Autodesk Fusion 360 part; units mm, degrees
sketch "Sketch1" plane through (0, 0, 0) normal (0, 0, 1) x (1, 0, 0)
  line L0 (-50, 25) -> (7.7, 25)
  line L1 (7.7, 25) -> (7.7, 7.3)
  line L2 (7.7, 7.3) -> (-50, 7.3)
  line L3 (-50, 7.3) -> (-50, 25)
  line L4 (6.7, 8.3) -> (-49, 8.3)
  line L5 (-49, 8.3) -> (-49, 24)
  line L6 (-49, 24) -> (6.7, 24)
  line L7 (6.7, 24) -> (6.7, 8.3)
  line L8 (6.7, 8.3) -> (-49, 24) construction
  line L9 (-49, 8.3) -> (6.7, 24) construction
  point P0 (-21.15, 16.15)
  dimension "d1" = 57.7
  dimension "d2" = 17.7
  dimension "d3" = 55.7
  dimension "d4" = 15.7
extrude "Extrude1" add sketch "Sketch1" along normal blind 2 contours L4 L5 L6 L7
extrude "Extrude2" add sketch "Sketch1" along normal blind 13
fillet "Fillet1" radius 2 4 edges at (7.7, 7.3, 6.5) (7.7, 25, 6.5) (-50, 7.3, 6.5) (-50, 25, 6.5)
fillet "Fillet2" radius 2 8 edges at (7.1142, 7.8858, 0) (-21.15, 7.3, 0) (-49.4142, 7.8858, 0) (-50, 16.15, 0) (-49.4142, 24.4142, 0) (-21.15, 25, 0) (7.1142, 24.4142, 0) (7.7, 16.15, 0)
Model file for the job. Use its own axes, mm. A direction names the side the tool comes from. Coordinates: 2 decimals unless noted, no trailing zeros. Loops run counter-clockwise (first coordinate to the right, second up) from the corner with the lowest first, then second, coordinate; pieces in that order, holes last. Notation, with made-up numbers: (-11, 65) - (35, 65) arc R21 cw to (35, 88) - close; hole circle Ø7 at (-17, -33.75). An arc over 180 degrees is marked (long way). Answer as a JSON object with one key per item and string values. Group by question number.
(1) Probe line 1 along Y through (x, z) = (0.5, 4); line 2 along X through (y, z) = (22.25, 4.5); line 3 along Z through (x, y) = (2.5, 16). List the from-to ranges inside material, lowest first.
(2) Cut at D-D (z = 1). Give the cut face in (x, y), then the cut area to 3 significant figures.
(3) Two-plate mould, pull along Y, no slides. Class faces 1 (the face through (-22, 16, 2)), 2 (the face through (-22, 25, 7)), 3 (the face through (-21, 7.3, 7)): released by +Y, released by -Y, zero draft, split by the parting line, or undercut.
(4) Cut at A-A (x = -17). Give the cut face in (y, z).
(5) Tool access for faces 4 (the face through (6.7, 16, 7)), 5 (the face through (-50, 16, 7)): list every direction of +Z, -Z, +X, -X, +Y, -Y with a clear straight run to the whole face (end or side of a thin tool).
(6) Flat gauge pin, fed straight in: pin 1 (1.5 mm diameter, centred on x = -11, y = 14, fed in from +Z). Where does the tip first touch, or does it go through?
(7) Cut at C-C (y = 21.5). Give the cut face in (x, z).
(8) Cut at B-B (z = 9.25). Give the cut face in (x, y).
Geometry says:
{
 "1": {"line 1": "y = 7.3 to 8.3, 24 to 25", "line 2": "x = -50 to -49, 6.7 to 7.7", "line 3": "z = 0 to 2"},
 "2": {"outline": "(-49.73, 9.3) arc R1.73 ccw to (-48, 7.57) - (5.7, 7.57) arc R1.73 ccw to (7.43, 9.3) - (7.43, 23) arc R1.73 ccw to (5.7, 24.73) - (-48, 24.73) arc R1.73 ccw to (-49.73, 23) - close", "area": "979 mm^2"},
 "3": {"face 1": "undercut", "face 2": "released by +Y", "face 3": "released by -Y"},
 "4": {"outline": "(7.3, 2) arc R2 ccw to (9.3, 0) - (23, 0) arc R2 ccw to (25, 2) - (25, 13) - (24, 13) - (24, 2) - (8.3, 2) - (8.3, 13) - (7.3, 13) - close"},
 "5": {"face 4": "+Z", "face 5": "+Z, -Z, -X, +Y, -Y"},
 "6": {"pin 1": "stops at z = 2"},
 "7": {"outline": "(-50, 2) arc R2 ccw to (-48, 0) - (5.7, 0) arc R2 ccw to (7.7, 2) - (7.7, 13) - (6.7, 13) - (6.7, 2) - (-49, 2) - (-49, 13) - (-50, 13) - close"},
 "8": {"outline": "(-50, 9.3) arc R2 ccw to (-48, 7.3) - (5.7, 7.3) arc R2 ccw to (7.7, 9.3) - (7.7, 23) arc R2 ccw to (5.7, 25) - (-48, 25) arc R2 ccw to (-50, 23) - close; hole (-49, 8.3) - (6.7, 8.3) - (6.7, 24) - (-49, 24) - close"}
}
